Check sheet for the modelled part. Datum: model origin and axes. Units: mm. Face numbers are marked on the shaded views. A direction names the side the tool comes from. Round coordinates to 2 decimals unless told otherwise and drop trailing zeros. Loops run counter-clockwise (first coordinate to the right, second up) from the corner with the lowest first, then second, coordinate; pieces in that order, holes last. Notation, with made-up numbers: M -19,83.5 L 13,83.5 A13 ccw 13,107.5 Z; hole C 20,48.5 d2. An arc over 180 degrees is marked long. One line per question, with ' | ' between items. Start each with the question number.
(1) Draft check along Y on the marked faces 1, 2 and 3. Enter one of: +Y half, -Y half, draft (parallel to the pull), parting line (faces both ways), or undercut.
(2) Thickness scan on probe 1 along Y at (x, z) = (0, 3); probe 2 along Y at (x, z) = (0, 9.7) (3 decimals); probe 3 along Z at (x, y) = (9.5, -5.5). Record the ranges inside material, lowest first. Write a range as [from, to].
(3) Section check D-D (z = 14.75). Record the boundary of the cut face in (x, y) (3 decimals), and give its area (3 significant figures).
(4) Section check A-A (x = 0). Record the boundary of the cut face in (y, z) (3 decimals), and give its area (3 significant figures).
(5) Go/stop test with flat-tipped pins: P1, Ø6, axis at x = 0, y = 0, coming from the +Z side; P2, Ø1.5, axis at y = -4, z = 7.5, coming from the +X side; P3, Ø6, axis at x = 6, z = 14.5, coming from the +Y side; P4, Ø8, axis at y = -2.5, z = 8, coming from the +X side. Record where each tip stops, or that it passes through.
(6) Tool access check on the marked faces 4, 5 and 6. Record the directions out of +Z, -Z, +X, -X, +Y, -Y that give a thin tool (end or side, any length) a straight path to the whole face; none if there is none.
(7) Section check C-C (z = 9). Record the boundary of the cut face in (x, y) (3 decimals).
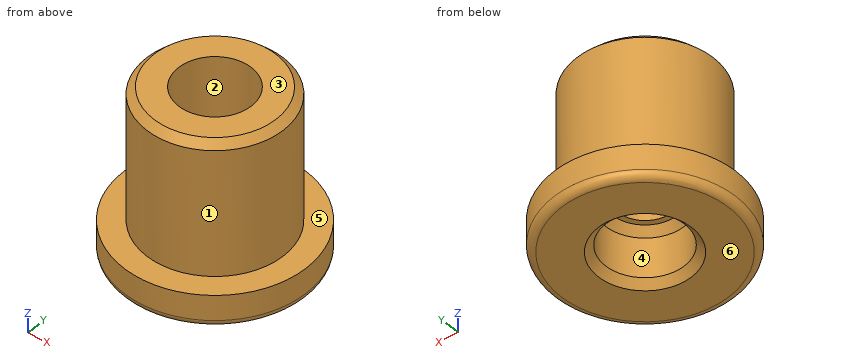
```python
from build123d import *

# Parameters (mm, degrees)
SKETCH_1_R          = 12.7
SKETCH_1_R_2        = 3.75
EXTRUDE_1_DEPTH     = 3
SKETCH_2_R          = 9.525
SKETCH_2_R_2        = 5.075
EXTRUDE_2_DEPTH     = 20
CHAMFER_1_SIZE      = 1
FILLET_1_R          = 1
SKETCH_3_R          = 12.7
SKETCH_3_R_2        = 9.525
EXTRUDE_3_DEPTH     = 1.5
SKETCH_4_R          = 5.075
SKETCH_4_R_2        = 3.75
EXTRUDE_4_DEPTH     = 7.8
SKETCH_5_R          = 5.5
CUT_EXTRUDE_1_DEPTH = 7.5
CHAMFER_2_SIZE      = 1


with BuildPart() as part:
    # 스케치1 → 보스-돌출1 (new body)
    with BuildSketch(Plane.XY):
        Circle(SKETCH_1_R)
        Circle(SKETCH_1_R_2, mode=Mode.SUBTRACT)
    extrude(amount=EXTRUDE_1_DEPTH)

    # 스케치2 → 보스-돌출2 (add)
    with BuildSketch(Plane.XY.offset(3)):
        Circle(SKETCH_2_R)
        Circle(SKETCH_2_R_2, mode=Mode.SUBTRACT)
    extrude(amount=EXTRUDE_2_DEPTH)

    # 모따기1
    chamfer_1_edges = [part.edges().sort_by_distance(p)[0] for p in [
        (-9.525, 0, 23),
    ]]
    chamfer(chamfer_1_edges, length=CHAMFER_1_SIZE)

    # 필렛1
    fillet_1_edges = [part.edges().sort_by_distance(p)[0] for p in [
        (-12.7, 0, 0),
    ]]
    fillet(fillet_1_edges, radius=FILLET_1_R)

    # 스케치3 → 보스-돌출3 (add)
    with BuildSketch(Plane.XY.offset(3)):
        Circle(SKETCH_3_R)
        Circle(SKETCH_3_R_2, mode=Mode.SUBTRACT)
    extrude(amount=EXTRUDE_3_DEPTH)

    # 스케치4 → 보스-돌출4 (add)
    with BuildSketch(Plane.XY.offset(3)):
        Circle(SKETCH_4_R)
        Circle(SKETCH_4_R_2, mode=Mode.SUBTRACT)
    extrude(amount=EXTRUDE_4_DEPTH)

    # 스케치5 → 컷-돌출1 (cut)
    with BuildSketch(Plane(origin=(0, 0, 0), x_dir=(-1, 0, 0), z_dir=(0, 0, -1))):
        Circle(SKETCH_5_R)
    extrude(amount=-CUT_EXTRUDE_1_DEPTH, mode=Mode.SUBTRACT)

    # 모따기2
    chamfer_2_edges = [part.edges().sort_by_distance(p)[0] for p in [
        (5.5, 0, 7.5),
        (5.5, 0, 0),
    ]]
    chamfer(chamfer_2_edges, length=CHAMFER_2_SIZE)


solid = part.part
```
The answers:
1) face 1: parting line | face 2: undercut | face 3: draft
2) probe 1: [-12.7, -5.5], [5.5, 12.7] | probe 2: [-9.525, -3.75], [3.75, 9.525] | probe 3: [0, 4.5]
3) outline: C 0,0 d19.05; hole C 0,0 d10.15 | area: 204 mm²
4) outline: M -12.7,1 A1 ccw -11.7,0 L -6.5,0 L -5.5,1 L -5.5,6.5 L -4.5,7.5 L -3.75,7.5 L -3.75,10.8 L -5.075,10.8 L -5.075,23 L -8.525,23 L -9.525,22 L -9.525,4.5 L -12.7,4.5 Z; M 3.75,7.5 L 4.5,7.5 L 5.5,6.5 L 5.5,1 L 6.5,0 L 11.7,0 A1 ccw 12.7,1 L 12.7,4.5 L 9.525,4.5 L 9.525,22 L 8.525,23 L 5.075,23 L 5.075,10.8 L 3.75,10.8 Z | area: 234 mm²
5) P1: through | P2: x = 8.95 | P3: y = 9.04 | P4: x = 12.69
6) face 4: -Z | face 5: +Z | face 6: -Z, +X, -X, +Y, -Y
7) outline: C 0,0 d19.05; hole C 0,0 d7.5
